Autodesk Fusion 360 part; units mm, degrees
sketch "Sketch1" plane through (0, 0, 0) normal (0, 1, 0) x (1, 0, 0) in component "Component"
  circle A0 centre (0, 0) radius 250
  dimension "d7" = 500
extrude "Extrude1" add sketch "Sketch1" along normal blind 1500 in component "Component"
sketch "Sketch2" plane through (0, 0, 0) normal (0, 0, 1) x (1, 0, 0) in component "Component"
  circle A0 centre (0, 175) radius 20
  line L0 (0, 0) -> (0, 1500) construction
  circle A1 centre (0, 875) radius 20
  dimension "d10" = 40
  dimension "d11" = 1500
  dimension "d13" = 175
  dimension "d14" = 40
  dimension "d15" = 700
extrude "Extrude2" cut sketch "Sketch2" along normal blind 475 in component "Component"
sketch "Sketch3" plane through (0, 0, 0) normal (0, -1, 0) x (1, 0, 0) in component "Component"
  circle A0 centre (0, 0) radius 250
  circle A1 centre (0, 0) radius 20
  dimension "d18" = 40
extrude "Extrude3" cut sketch "Sketch3" against normal blind 1700 contours A1 in component "Component"
component "Component" placed x (1, 0, 0) y (0, 1, 0) z (0, 0, 1) at (0, 0, 0)
Geometry: final body of the model. Coordinates: model frame, mm. A direction names the side the tool comes from. Round coordinates to 2 decimals unless told otherwise and drop trailing zeros. Loops run counter-clockwise (first coordinate to the right, second up) from the corner with the lowest first, then second, coordinate; pieces in that order, holes last. Notation, with made-up numbers: (5, 65.25) -> (14, 65.25) arc R13 cw to (14, 88.25) -> close; hole circle Ø10 at (-38.75, -32.5). An arc over 180 degrees is marked (long way). One line per question, with ' | ' between items. Start each with the question number.
1. Set-up query: faces 1 (the face through (19.076, 868.993, 123.25)), 2 (the face through (-3, 1500, 52)). Return all of +Z, -Z, +X, -X, +Y, -Y with unobstructed straight access to the full face (end or side cutting, diameter ignored); none if empty.
2. Line query: line 1 along Y through (x, z) = (0, 173); line 2 along X through (y, z) = (486, 0); line 3 along Y through (x, z) = (7, 65) (3 decimals). Output: solid intervals per line, ascending. Write a range as [from, to].
3. Section A-A on x = 0. Output: boundary loops of the cut face in (y, z).
4. Section C-C on z = 152. Output: boundary loops of the cut face in (x, y).
5. Mould query, pull axis X, two halves, no side actions, for faces 3 (the face through (-249.76, 739.5, 10.99)), 4 (the face through (-3, 0, 52)), 5 (the face through (19.076, 168.993, 123.25)). Classes: pulls with the +X half, pulls with the -X half, needs draft (parallel to the pull), parting line crosses it, or undercut.
6. Contact query for flat-ended pins moving along their axis: pin 1 (3 mm diameter, centred on y = 1309.5, z = -166.5, fed in from +X); pin 2 (2 mm diameter, centred on y = 473.5, z = -141.5, fed in from -X); pin 3 (1 mm diameter, centred on x = 4.5, y = 880, fed in from +Z); pin 4 (1.5 mm diameter, centred on x = 177.5, z = 23.5, fed in from -Y). Output: stop coordinate, or through.
7. Section B-B on y = 529. Output: boundary loops of the cut face in (x, z), and give its area (3 significant figures).
8. Section D-D on y = 875. Output: boundary loops of the cut face in (x, z), and give its area (3 significant figures).
Returned:
1) face 1: +Z | face 2: +Z, -Z, +X, -X, +Y
2) line 1: y = [0, 155], [195, 855], [895, 1500] | line 2: x = [-250, -20], [20, 250] | line 3: y = [0, 156.265], [193.735, 856.265], [893.735, 1500]
3) outline: (0, -250) -> (1500, -250) -> (1500, -20) -> (0, -20) -> close; (0, 20) -> (155, 20) -> (155, 250) -> (0, 250) -> close; (195, 20) -> (855, 20) -> (855, 250) -> (195, 250) -> close; (895, 20) -> (1500, 20) -> (1500, 250) -> (895, 250) -> close
4) outline: (-198.48, 0) -> (198.48, 0) -> (198.48, 1500) -> (-198.48, 1500) -> close; hole circle Ø40 at (0, 175); hole circle Ø40 at (0, 875)
5) face 3: parting line crosses it | face 4: needs draft | face 5: undercut
6) pin 1: stops at x = 187.82 | pin 2: stops at x = -206.78 | pin 3: stops at z = -19.36 | pin 4: stops at y = 0
7) outline: circle Ø500 at (0, 0); hole circle Ø40 at (0, 0) | area: 195,000 mm2
8) outline: (-20, 0) -> (-20, 249.2) arc R250 ccw (long way) to (20, 249.2) -> (20, 0) arc R20 cw to start | area: 186,000 mm2
